Design review of the part built by this model. Coordinates are the model's own, in mm. A direction names the side the tool comes from. Coordinates: 2 decimals unless noted, no trailing zeros. Loops run counter-clockwise (first coordinate to the right, second up) from the corner with the lowest first, then second, coordinate; pieces in that order, holes last. Notation, with made-up numbers: (-23, 55) - (26, 55) arc R16 cw to (26, 72) - close; hole circle Ø1 at (41.5, -31). An arc over 180 degrees is marked (long way). Use one line per item in the form item = value. Start each with the question number.
(1) Add section D-D (z = 2.25). Count the separate pieces of the cut face and the enclosed holes in it, plus the area to 3 significant figures.
(2) For L1, parallel to Y at x = -20, z = 5; L2, parallel to Y at x = 40, z = 7.25; L3, parallel to Y at x = -8.5, z = 5, list the stretches that pass through material, from the lowest coordinate up.
(3) Add section B-B (z = 11.5). State the section outline as (x, y) points.
(4) Add section A-A (y = 0). State the section outline as (x, z) points, plus the area to 3 significant figures.
(5) Clearance check with flat-ended pins moving along their axes: pin 1 Ø2.5 at (x, y) = (-40, 0) entering from -Z; pin 2 Ø6 at (x, y) = (20, -25) entering from +Z; pin 3 Ø3 at (y, z) = (3.5, 14.5) entering from -X; pin 4 Ø2 at (x, z) = (-4, 12.5) entering from -Y. State where each tip first meets the part, or that it passes through.
(6) The part is to be moulded in two halves that separate along X. For faces 6 (the face through (39.512, 22.804, 5.07)), 7 (the face through (-1, 32.5, 5)), 8 (the face through (47.5, 0, 5)), say which applies: pulls with the +X half, pulls with the -X half, needs draft (parallel to the pull), parting line crosses it, or undercut.
(7) Tool access review of faces 1 (the face through (-1, -21, 0)), 2 (the face through (-30, 0, 8)), 3 (the face through (-30.361, -15.245, 13.204)), 4 (the face through (32.5, 0, 13)), 5 (the face through (-47.5, 0, 5)): name each direction out of +Z, -Z, +X, -X, +Y, -Y from which nothing blocks a thin tool from reaching the whole face with its end or side.
(8) Add section C-C (x = -20). State the section outline as (y, z) points.
```python
from build123d import *

# Parameters (mm, degrees)
F0_W     = 95
F0_H     = 65
F1_DEPTH = 10
F3_DEPTH = 7.5
F4_R     = 1
F6_DEPTH = 10.001
F7_R     = 2.25
F8_DEPTH = 10.001


with BuildPart() as f1:
    # F0 (on Top) → F1 (new body)
    with BuildSketch(Plane.XY):
        Rectangle(F0_W, F0_H)
    extrude(amount=F1_DEPTH)

    # F2 (on face) → F3 (join)
    with BuildSketch(Plane.XY.offset(10)):
        with BuildLine():
            Line((32.5, -10), (32.5, 10))
            ThreePointArc((32.5, 10), (30.303301, 15.303301), (25, 17.5))
            Line((25, 17.5), (-25, 17.5))
            ThreePointArc((-25, 17.5), (-30.303301, 15.303301), (-32.5, 10))
            Line((-32.5, 10), (-32.5, -10))
            ThreePointArc((-32.5, -10), (-30.303301, -15.303301), (-25, -17.5))
            Line((-25, -17.5), (25, -17.5))
            ThreePointArc((25, -17.5), (30.303301, -15.303301), (32.5, -10))
        make_face()
        with BuildLine():
            ThreePointArc((30, -10), (28.535534, -13.535534), (25, -15))
            Line((25, -15), (-25, -15))
            ThreePointArc((-25, -15), (-28.535534, -13.535534), (-30, -10))
            Line((-30, -10), (-30, 10))
            ThreePointArc((-30, 10), (-28.535534, 13.535534), (-25, 15))
            Line((-25, 15), (25, 15))
            ThreePointArc((25, 15), (28.535534, 13.535534), (30, 10))
            Line((30, 10), (30, -10))
        make_face(mode=Mode.SUBTRACT)
    extrude(amount=F3_DEPTH)

    # F4
    f4_edges = [f1.edges().sort_by_distance(p)[0] for p in [
        (32.5, 0, 17.5),
        (30.303301, 15.303301, 17.5),
        (0, 17.5, 17.5),
        (-30.303301, 15.303301, 17.5),
        (-32.5, 0, 17.5),
        (-30.303301, -15.303301, 17.5),
        (0, -17.5, 17.5),
        (30.303301, -15.303301, 17.5),
        (28.535534, -13.535534, 17.5),
        (0, -15, 17.5),
        (-28.535534, -13.535534, 17.5),
        (-30, 0, 17.5),
        (-28.535534, 13.535534, 17.5),
        (0, 15, 17.5),
        (28.535534, 13.535534, 17.5),
        (30, 0, 17.5),
    ]]
    fillet(f4_edges, radius=F4_R)

    # F5 (on face) → F6 (cut, through all)
    with BuildSketch(Plane.XY.offset(10)):
        with BuildLine():
            Line((-25, -15), (25, -15))
            ThreePointArc((25, -15), (28.535534, -13.535534), (30, -10))
            Line((30, -10), (30, 10))
            ThreePointArc((30, 10), (28.535534, 13.535534), (25, 15))
            Line((25, 15), (-25, 15))
            ThreePointArc((-25, 15), (-28.535534, 13.535534), (-30, 10))
            Line((-30, 10), (-30, -10))
            ThreePointArc((-30, -10), (-28.535534, -13.535534), (-25, -15))
        make_face()
    extrude(amount=-F6_DEPTH, mode=Mode.SUBTRACT)

    # F7 (on face) → F8 (cut, through all)
    with BuildSketch(Plane.XY.offset(10)):
        with Locations((-40, 25)):
            Circle(F7_R)
        with Locations((-40, 0)):
            Circle(F7_R)
        with Locations((-40, -25)):
            Circle(F7_R)
        with Locations((-20, 25)):
            Circle(F7_R)
        with Locations((-20, -25)):
            Circle(F7_R)
        with Locations((0, 25)):
            Circle(F7_R)
        with Locations((0, -25)):
            Circle(F7_R)
        with Locations((20, 25)):
            Circle(F7_R)
        with Locations((20, -25)):
            Circle(F7_R)
        with Locations((40, 25)):
            Circle(F7_R)
        with Locations((40, 0)):
            Circle(F7_R)
        with Locations((40, -25)):
            Circle(F7_R)
    extrude(amount=-F8_DEPTH, mode=Mode.SUBTRACT)


solid = f1.part
```
Computed values:
q1.separate_pieces = 1
q1.enclosed_holes = 13
q1.area = 4,210 mm^2
q2.L1 = -32.5 to -27.25, -22.75 to -15, 15 to 22.75, 27.25 to 32.5
q2.L2 = -32.5 to -27.25, -22.75 to -2.25, 2.25 to 22.75, 27.25 to 32.5
q2.L3 = -32.5 to -15, 15 to 32.5
q3.outline = (-32.5, -10) arc R7.5 ccw to (-25, -17.5) - (25, -17.5) arc R7.5 ccw to (32.5, -10) - (32.5, 10) arc R7.5 ccw to (25, 17.5) - (-25, 17.5) arc R7.5 ccw to (-32.5, 10) - close; hole (-30, -10) arc R5 ccw to (-25, -15) - (25, -15) arc R5 ccw to (30, -10) - (30, 10) arc R5 ccw to (25, 15) - (-25, 15) arc R5 ccw to (-30, 10) - close
q4.outline = (-47.5, 0) - (-42.25, 0) - (-42.25, 10) - (-47.5, 10) - close; (-37.75, 0) - (-30, 0) - (-30, 16.5) arc R1 ccw to (-31, 17.5) - (-31.5, 17.5) arc R1 ccw to (-32.5, 16.5) - (-32.5, 10) - (-37.75, 10) - close; (30, 0) - (37.75, 0) - (37.75, 10) - (32.5, 10) - (32.5, 16.5) arc R1 ccw to (31.5, 17.5) - (31, 17.5) arc R1 ccw to (30, 16.5) - close; (42.25, 0) - (47.5, 0) - (47.5, 10) - (42.25, 10) - close
q4.area = 297 mm^2
q5.pin_1 = through
q5.pin_2 = 10
q5.pin_3 = -32.5
q5.pin_4 = -17.5
q6.face_6 = undercut
q6.face_7 = needs draft
q6.face_8 = pulls with the +X half
q7.face_1 = -Z, +X, -X, +Y, -Y
q7.face_2 = +Z, -Z
q7.face_3 = +Z, -X, -Y
q7.face_4 = +Z, +X, +Y, -Y
q7.face_5 = +Z, -Z, -X, +Y, -Y
q8.outline = (-32.5, 0) - (-27.25, 0) - (-27.25, 10) - (-32.5, 10) - close; (-22.75, 0) - (-15, 0) - (-15, 16.5) arc R1 ccw to (-16, 17.5) - (-16.5, 17.5) arc R1 ccw to (-17.5, 16.5) - (-17.5, 10) - (-22.75, 10) - close; (15, 0) - (22.75, 0) - (22.75, 10) - (17.5, 10) - (17.5, 16.5) arc R1 ccw to (16.5, 17.5) - (16, 17.5) arc R1 ccw to (15, 16.5) - close; (27.25, 0) - (32.5, 0) - (32.5, 10) - (27.25, 10) - close
